Answer from the drawing. Dimensions are ordinates in mm from the lowest x, y and z of the part. Coordinates: 2 decimals unless noted, no trailing zeros. Loops run counter-clockwise (first coordinate to the right, second up) from the corner with the lowest first, then second, coordinate; pieces in that order, holes last. Notation, with made-up numbers: (4, 6) - (33, 6) arc R9 ccw to (33, 22) - close; hole circle Ø5 at (-2, 0.5). An arc over 180 degrees is marked (long way). Use one line per item in the form item = value. Start each with the question number.
1) A cutting plane is placed at A-A (x = 10). Give the vertices of the cut face in (y, z).
2) A cutting plane is placed at C-C (y = 28.5). State how many separate pieces and enclosed holes the cut face has, and give its area (3 significant figures).
3) Consider line 1 (X direction, y = 44.5, z = 6); line 2 (Y direction, x = 30, z = 11.3); line 3 (X direction, y = 12, z = 8.75). Determine where each line is inside the solid, lowest interval first.
4) The mould has two halves that part along X. Classify the marked faces 1, 2, 3 and 4: released by +X, released by -X, zero draft, split by the parting line, or undercut.
5) Each of these flat-tipped pins is pushed along its axis until it touches: P1, Ø8.5, axis at x = 70, y = 30, coming from the +Z side; P2, Ø13, axis at x = 40, y = 32.4, coming from the -Z side. Where does it stop, or does it pass through?
6) A cutting plane is placed at B-B (z = 2.25). Give the vertices of the cut face in (x, y), and give its area (3 significant figures).
7) A cutting plane is placed at D-D (y = 10). Give the vertices of the cut face in (x, z), and give its area (3 significant figures).
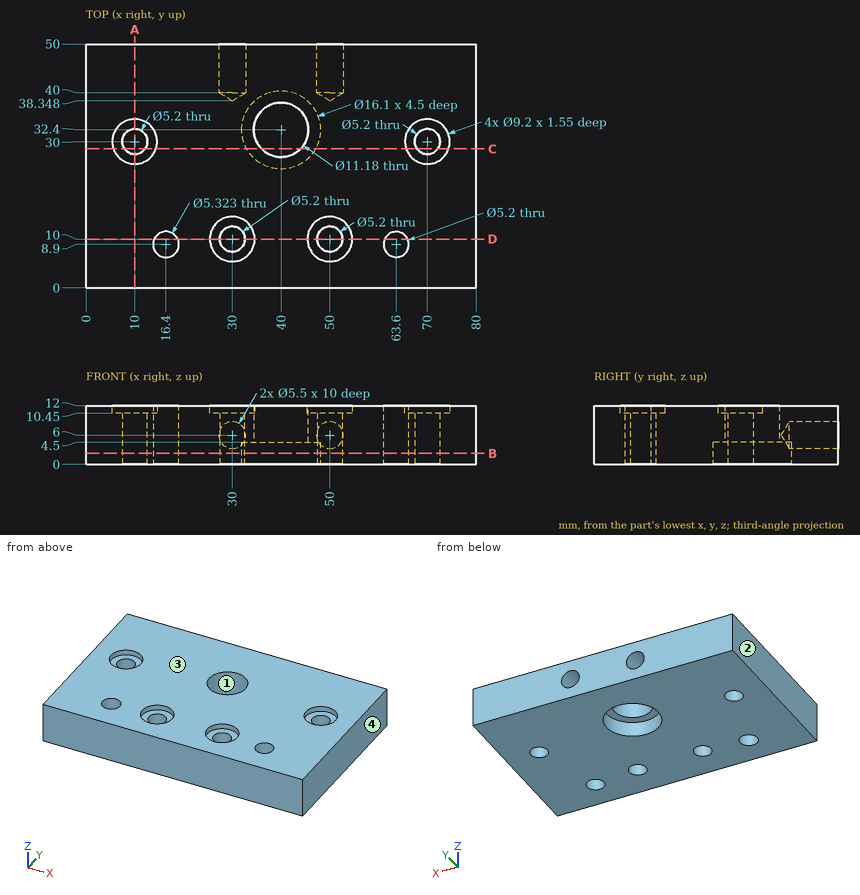
Found:
q1.outline = (0, 0) - (27.4, 0) - (27.4, 10.45) - (25.4, 10.45) - (25.4, 12) - (0, 12) - close; (32.6, 0) - (50, 0) - (50, 12) - (34.6, 12) - (34.6, 10.45) - (32.6, 10.45) - close
q2.separate_pieces = 4
q2.enclosed_holes = 0
q2.area = 721 mm^2
q3.line_1 = 0 to 27.25, 32.75 to 47.25, 52.75 to 80
q3.line_2 = 0 to 5.4, 14.6 to 50
q3.line_3 = 0 to 28.34, 31.66 to 48.34, 51.66 to 80
q4.face_1 = undercut
q4.face_2 = released by -X
q4.face_3 = zero draft
q4.face_4 = released by +X
q5.P1 = 10.45
q5.P2 = 4.5
q6.outline = (0, 0) - (80, 0) - (80, 50) - (0, 50) - close; hole circle Ø5.2 at (10, 30); hole circle Ø5.32 at (16.4, 8.9); hole circle Ø5.2 at (30, 10); hole circle Ø16.1 at (40, 32.4); hole circle Ø5.2 at (50, 10); hole circle Ø5.2 at (63.6, 8.9); hole circle Ø5.2 at (70, 30)
q6.area = 3,670 mm^2
q7.outline = (0, 0) - (13.98, 0) - (13.98, 12) - (0, 12) - close; (18.82, 0) - (27.4, 0) - (27.4, 10.45) - (25.4, 10.45) - (25.4, 12) - (18.82, 12) - close; (32.6, 0) - (47.4, 0) - (47.4, 10.45) - (45.4, 10.45) - (45.4, 12) - (34.6, 12) - (34.6, 10.45) - (32.6, 10.45) - close; (52.6, 0) - (61.24, 0) - (61.24, 12) - (54.6, 12) - (54.6, 10.45) - (52.6, 10.45) - close; (65.96, 0) - (80, 0) - (80, 12) - (65.96, 12) - close
q7.area = 708 mm^2
